Read the model definition and answer for the solid it produces. Units are mm, in the model's axes. A direction names the side the tool comes from. Coordinates: 2 decimals unless noted, no trailing zeros. Loops run counter-clockwise (first coordinate to the right, second up) from the corner with the lowest first, then second, coordinate; pieces in that order, holes last.
from build123d import *

# Parameters (mm, degrees)
SKETCH2_R           = 7.5
ROTAITING_PIN_DEPTH = 30
BODY_DEPTH          = 15
SKETCH4_R           = 7.5
HOLE_DEPTH          = 30


with BuildPart() as part:
    # Sketch2 → rotaiting pin (new body)
    with BuildSketch(Plane(origin=(0, 0, 0), x_dir=(1, 0, 0), z_dir=(0, 1, 0))):
        with Locations(Location((0, 0, 0), (0, 0, 270))):
            Circle(SKETCH2_R)
    extrude(amount=ROTAITING_PIN_DEPTH)

    # Sketch3 → body (add, symmetric)
    with BuildSketch(Plane.XY):
        Polygon((-17.5, 60), (-7.5, 60), (-7.5, 40), (12.5, 40), (12.5, 30), (-17.5, 30), align=None)
    extrude(amount=BODY_DEPTH, both=True)

    # Sketch4 → hole (cut)
    with BuildSketch(Plane(origin=(-7.5, 0, 0), x_dir=(0, 0, -1), z_dir=(1, 0, 0))):
        with Locations(Location((0, 50, 0), (0, 0, 90))):
            Circle(SKETCH4_R)
    extrude(amount=-HOLE_DEPTH, mode=Mode.SUBTRACT)


solid = part.part
Q1. Determine the mould class of faces 1 (the face through (-12.43, 54.032, 6.324)), 2 (the face through (-13, 60, 0)), 3 (the face through (0, 0, 0)) for opening direction Y: +Y half, -Y half, draft (parallel to the pull), parting line (faces both ways), or undercut.
Findings below:
face 1: undercut
face 2: +Y half
face 3: -Y half
Q2. Straight lines are drawn through the part: probe 1 along Z at (x, y) = (-15.5, 50); probe 2 along Y at (x, z) = (4.5, 7); probe 3 along Y at (x, z) = (-15, 6). For each, find the intervals that lie inside material, in ascending order.
Findings below:
probe 1: z = -15 to -7.5, 7.5 to 15
probe 2: y = 30 to 40
probe 3: y = 30 to 45.5, 54.5 to 60
Q3. A cutting plane is placed at C-C (x = -12). Give the vertices of the cut face in (y, z), then the cut area to 3 significant figures.
Findings below:
outline: (30, -15) - (60, -15) - (60, 15) - (30, 15) - close; hole circle Ø15 at (50, 0)
area: 723 mm2
Q4. Flat-ended cylindrical pins translate along their axes: pin 1 Ø2 at (x, z) = (-2, -6.5) entering from +Y; pin 2 Ø3 at (y, z) = (22.5, 7.5) entering from -X; pin 3 Ø1.5 at (x, z) = (-5.5, -7.5) entering from -Y. Find the tip coordinate at first contact, or state that the pin passes through.
Findings below:
pin 1: stops at y = 40
pin 2: stops at x = -4.5
pin 3: stops at y = 30
Q5. A cutting plane is placed at A-A (z = 0). Give the vertices of the cut face in (x, y).
Findings below:
outline: (-17.5, 30) - (-7.5, 30) - (-7.5, 0) - (7.5, 0) - (7.5, 30) - (12.5, 30) - (12.5, 40) - (-7.5, 40) - (-7.5, 42.5) - (-17.5, 42.5) - close; (-17.5, 57.5) - (-7.5, 57.5) - (-7.5, 60) - (-17.5, 60) - close
Q6. A cutting plane is placed at B-B (y = 45.5). Give the vertices of the cut face in (x, z), then the cut area to 3 significant figures.
Findings below:
outline: (-17.5, -15) - (-7.5, -15) - (-7.5, -6) - (-17.5, -6) - close; (-17.5, 6) - (-7.5, 6) - (-7.5, 15) - (-17.5, 15) - close
area: 180 mm2
Q7. Which of the six approach directions +Z, -Z, +X, -X, +Y, -Y give full straight-line access (tool end or side, diameter ignored) to faces 4 (the face through (-9, 30, 0)), 5 (the face through (2, 40, 0)), 6 (the face through (-17.5, 41, 0))?
Findings below:
face 4: -Y
face 5: +Z, -Z, +X, +Y
face 6: +Z, -Z, -X, +Y, -Y
Q8. A cutting plane is placed at D-D (x = 0). Give the vertices of the cut face in (y, z).
Findings below:
outline: (0, -7.5) - (30, -7.5) - (30, -15) - (40, -15) - (40, 15) - (30, 15) - (30, 7.5) - (0, 7.5) - close
